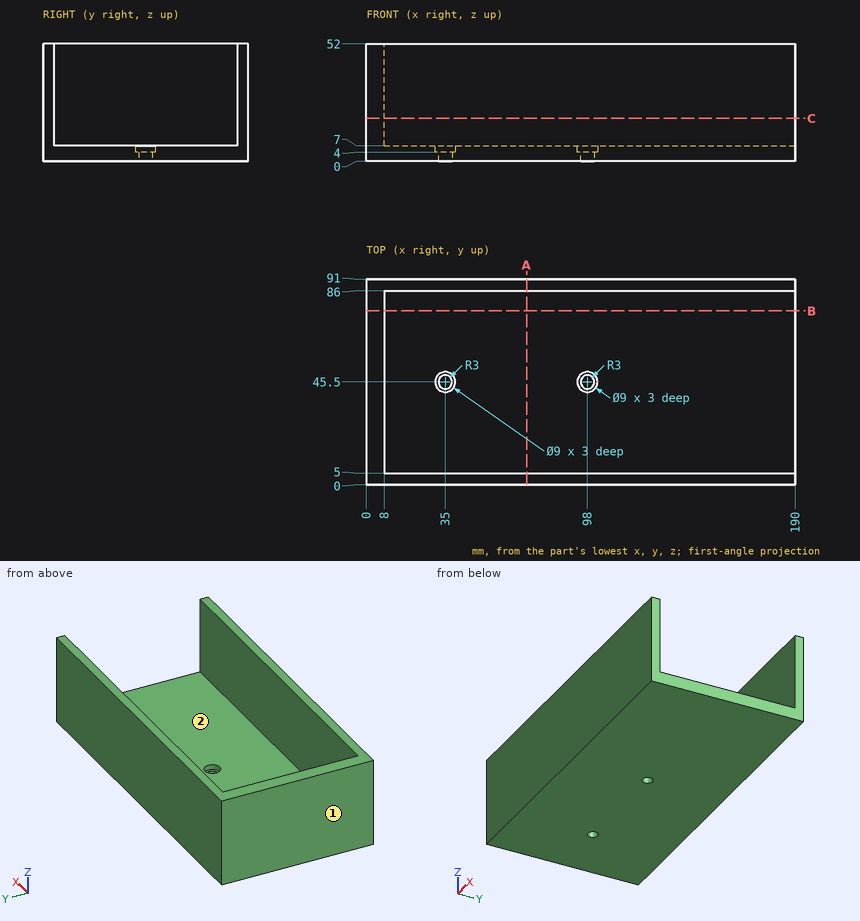
For this review, use the dimensioned drawing (mm, ordinates from the lowest corner) and the shaded views. A direction names the side the tool comes from. Coordinates: 2 decimals unless noted, no trailing zeros. Loops run counter-clockwise (first coordinate to the right, second up) from the corner with the lowest first, then second, coordinate; pieces in that order, holes last.
1. For the marked faces 1 and 2, list the 3-axis set-ups (+Z, -Z, +X, -X, +Y, -Y) from which the entire face can be reached by the end or side of a thin tool; tool diameter is ignored.
2. Add section A-A, the plane x = 71. Give the boundary of the cut face in (y, z).
3. Add section C-C, the plane z = 19. Give the boundary of the cut face in (x, y).
4. For line 1 (Y direction, x = 178.5, z = 31); line 2 (X direction, y = 47, z = 4.5); line 3 (Y direction, x = 98, z = 5.2), list the stretches that pass through material, from the lowest coordinate up.
5. Insertion check: P1, Ø2.5, axis at x = 97.5, y = 46.5, coming from the +Z side; P2, Ø10.5, axis at x = 98, y = 45.5, coming from the -Z side; P3, Ø1.5, axis at x = 75.5, y = 67, coming from the +Z side; P4, Ø7, axis at x = 35, y = 45.5, coming from the +Z side. Each pin has a flat end and moves straight along its axis. Give the tip position at first contact, or say it passes through.
6. Add section B-B, the plane y = 77. Give the boundary of the cut face in (x, z).
Result:
1. face 1: +Z, -Z, -X, +Y, -Y
1. face 2: +Z, +X
2. outline: (0, 0) - (91, 0) - (91, 52) - (86, 52) - (86, 7) - (5, 7) - (5, 52) - (0, 52) - close
3. outline: (0, 0) - (190, 0) - (190, 5) - (8, 5) - (8, 86) - (190, 86) - (190, 91) - (0, 91) - close
4. line 1: y = 0 to 5, 86 to 91
4. line 2: x = 0 to 30.76, 39.24 to 93.76, 102.24 to 190
4. line 3: y = 0 to 41, 50 to 91
5. P1: passes through
5. P2: stops at z = 0
5. P3: stops at z = 7
5. P4: stops at z = 4
6. outline: (0, 0) - (190, 0) - (190, 7) - (8, 7) - (8, 52) - (0, 52) - close
